Geometry check sheet. Reference: drawing and pictorial views, mm from the part's lowest x, y, z. A direction names the side the tool comes from. Give positions to 0.01 mm unless a question says otherwise; leave off trailing zeros. Order: outer loops, then holes, each group sorted by start corner. A loop starts at its lowest first (then second) coordinate and runs counter-clockwise, first axis right, second up.
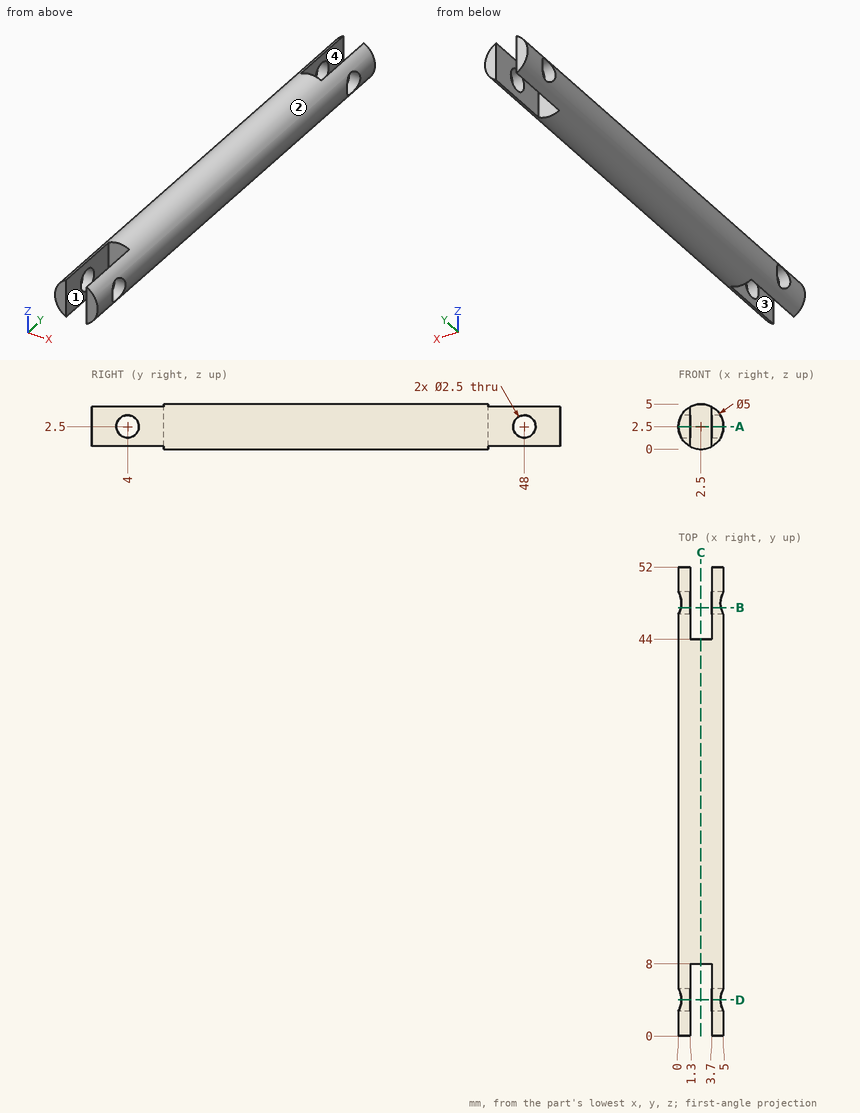
(1) Cross-section at D-D on y = 4. Enter the section's corners in (x, z), then the cut area to 3 significant figures.
Response values:
outline: (0.33, 1.25) arc R2.5 ccw to (1.3, 0.31) - (1.3, 1.25) - close; (0.33, 3.75) - (1.3, 3.75) - (1.3, 4.69) arc R2.5 ccw to start; (3.7, 0.31) arc R2.5 ccw to (4.67, 1.25) - (3.7, 1.25) - close; (3.7, 3.75) - (4.67, 3.75) arc R2.5 ccw to (3.7, 4.69) - close
area: 2.16 mm2
(2) Release check for a two-part mould opening along X. For the marked faces 1 and 2 record: released by +X, released by -X, zero draft, split by the parting line, or undercut.
Response values:
face 1: undercut
face 2: split by the parting line
(3) Cross-section at B-B on y = 47.5. Enter the section's corners in (x, z).
Response values:
outline: (0.28, 1.35) arc R2.5 ccw to (1.3, 0.31) - (1.3, 1.35) - close; (0.28, 3.65) - (1.3, 3.65) - (1.3, 4.69) arc R2.5 ccw to start; (3.7, 0.31) arc R2.5 ccw to (4.72, 1.35) - (3.7, 1.35) - close; (3.7, 3.65) - (4.72, 3.65) arc R2.5 ccw to (3.7, 4.69) - close
(4) Gauge pin test, flat ends, axial feed: pin 1 Ø2 at (y, z) = (48, 2.5) entering from +X; pin 2 Ø2 at (x, y) = (3, 46) entering from -Z; pin 3 Ø3 at (y, z) = (16.5, 4) entering from +X; pin 4 Ø1.2 at (x, z) = (2.5, 2.5) entering from -Y. Record the tip position at first contact, or that the pin passes through.
Response values:
pin 1: passes through
pin 2: stops at z = 0.31
pin 3: stops at x = 5
pin 4: stops at y = 8
(5) Cross-section at A-A on z = 2.5. Enter the section's corners in (x, y), then the cut area to 3 significant figures.
Response values:
outline: (0, 0) - (1.3, 0) - (1.3, 2.75) - (0, 2.75) - close; (0, 5.25) - (1.3, 5.25) - (1.3, 8) - (3.7, 8) - (3.7, 5.25) - (5, 5.25) - (5, 46.75) - (3.7, 46.75) - (3.7, 44) - (1.3, 44) - (1.3, 46.75) - (0, 46.75) - close; (0, 49.25) - (1.3, 49.25) - (1.3, 52) - (0, 52) - close; (3.7, 0) - (5, 0) - (5, 2.75) - (3.7, 2.75) - close; (3.7, 49.25) - (5, 49.25) - (5, 52) - (3.7, 52) - close
area: 209 mm2
(6) Material ranges on L1, parallel to Y at x = 4.65, z = 2.5; L2, parallel to Y at x = 4.45, z = 1.95; L3, parallel to Y at x = 2.05, z = 3.3, recorded low to high.
Response values:
L1: y = 0 to 2.75, 5.25 to 46.75, 49.25 to 52
L2: y = 0 to 2.88, 5.12 to 46.88, 49.12 to 52
L3: y = 8 to 44
(7) Set-up check for the marked faces 3 and 4: record each of +Z, -Z, +X, -X, +Y, -Y from which the full face is reachable in a straight line by a thin tool's end or side.
Response values:
face 3: +Z, -Z, -Y
face 4: +Z, -Z, +Y
(8) Cross-section at C-C on x = 2.5. Enter the section's corners in (y, z).
Response values:
outline: (8, 0) - (44, 0) - (44, 5) - (8, 5) - close
